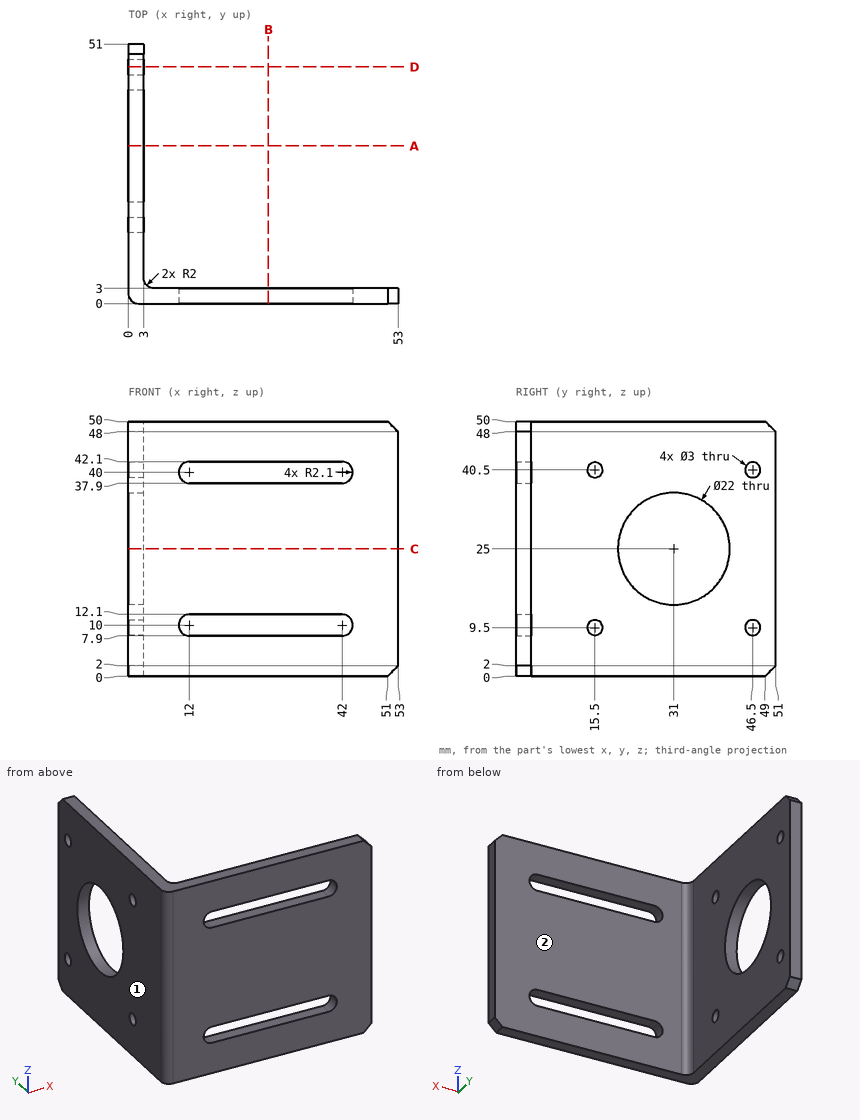
Verification items for this drawing (mm, ordinates from the low corner). A direction names the side the tool comes from. Give positions to 0.01 mm unless a question says otherwise; leave off trailing zeros. Loops run counter-clockwise (first coordinate to the right, second up) from the corner with the lowest first, then second, coordinate; pieces in that order, holes last.
(1) Section check A-A on y = 31. Record the cut outline in (x, z), then the cut area to 3 significant figures.
From the geometry:
outline: (0, 0) - (3, 0) - (3, 14) - (0, 14) - close; (0, 36) - (3, 36) - (3, 50) - (0, 50) - close
area: 84.0 mm2
(2) Section check D-D on y = 46.5. Record the cut outline in (x, z).
From the geometry:
outline: (0, 0) - (3, 0) - (3, 8) - (0, 8) - close; (0, 11) - (3, 11) - (3, 39) - (0, 39) - close; (0, 42) - (3, 42) - (3, 50) - (0, 50) - close
(3) Thickness scan on L1, parallel to Y at x = 2.4, z = 9.5; L2, parallel to Z at x = 2, y = 15; L3, parallel to Y at x = 24.5, z = 22.5. Record the ranges inside material, lowest first.
From the geometry:
L1: y = 0 to 14, 17 to 45, 48 to 51
L2: z = 0 to 8.09, 10.91 to 39.09, 41.91 to 50
L3: y = 0 to 3
(4) Set-up check for the marked faces 1 and 2: record each of +Z, -Z, +X, -X, +Y, -Y from which the full face is reachable in a straight line by a thin tool's end or side.
From the geometry:
face 1: +Z, -Z, -X, +Y, -Y
face 2: +Z, -Z, +X, +Y
(5) Section check B-B on x = 27.5. Record the cut outline in (y, z).
From the geometry:
outline: (0, 0) - (3, 0) - (3, 7.9) - (0, 7.9) - close; (0, 12.1) - (3, 12.1) - (3, 37.9) - (0, 37.9) - close; (0, 42.1) - (3, 42.1) - (3, 50) - (0, 50) - close
(6) Section check C-C on z = 25. Record the cut outline in (x, y), then the cut area to 3 significant figures.
From the geometry:
outline: (0, 2) arc R2 ccw to (2, 0) - (53, 0) - (53, 3) - (5, 3) arc R2 cw to (3, 5) - (3, 20) - (0, 20) - close; (0, 42) - (3, 42) - (3, 51) - (0, 51) - close
area: 237 mm2
(7) Depth check by flat-ended pin: pin 1 Ø2.5 at (y, z) = (15.5, 40.5) entering from -X; pin 2 Ø23 at (y, z) = (24.5, 30.5) entering from +X; pin 3 Ø10 at (x, z) = (42.5, 25) entering from +Y. Enter the tip coordinate at first touch or a pass-through.
From the geometry:
pin 1: passes through
pin 2: stops at x = 3
pin 3: stops at y = 3
